Job drawing, mm, ordinate dimensions from the low corner. One solid piece. A direction names the side the tool comes from. Give positions to 0.01 mm unless a question says otherwise; leave off trailing zeros. Order: outer loops, then holes, each group sorted by start corner. A loop starts at its lowest first (then second) coordinate and runs counter-clockwise, first axis right, second up. Notation, with made-up numbers: M 13,-12 L 57,-12 A31 ccw 57,23 Z; hole C -30.5,-17.75 d2. An arc over 180 degrees is marked long. Put each result on its own line as item: value. Start each with the question number.
1) Drill centre lines: line 1 (Z direction, x = 32, y = 34); line 2 (Y direction, x = 9.5, z = 55.5); line 3 (Y direction, x = 50, z = 1.8). Where is each one in solid material? Low to high. Write a range as [from, to].
2) Tool access for the marked faces 1 and 2: list every direction of +Z, -Z, +X, -X, +Y, -Y with a clear straight run to the whole face (end or side of a thin tool).
3) Cut at B-B (y = 35.5). Write the cut outline in (x, z).
4) Pin check, flat tips, straight feed: pin 1 (12 mm diameter, centred on x = 75.5, z = 104.5, fed in from +Y); pin 2 (5.5 mm diameter, centred on y = 9, z = 115, fed in from -X); pin 3 (5.5 mm diameter, centred on y = 4.5, z = 114.5, fed in from +X). Stop position of each tip, or through.
5) Cut at D-D (y = 61). Write the cut outline in (x, z).
6) Cut at A-A (x = 75). Write the cut outline in (y, z).
7) Cut at C-C (z = 44.5). Write the cut outline in (x, y), and give its area (3 significant figures).
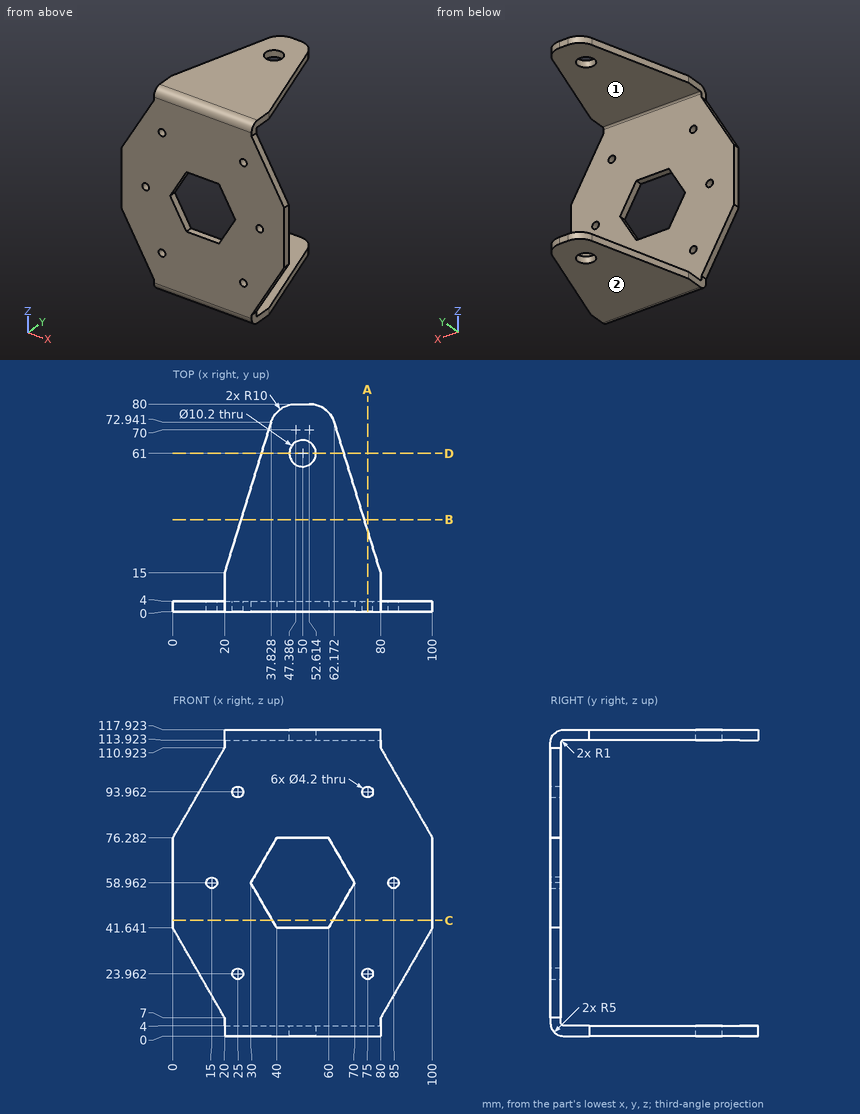
Solution:
1. line 1: [0, 4], [113.92, 117.92]
1. line 2: [0, 4]
1. line 3: [1.16, 55.9], [66.1, 80]
2. face 1: +X, -X, +Y
2. face 2: -Z, +X, -X, +Y, -Y
3. outline: M 26.31,0 L 73.69,0 L 73.69,4 L 26.31,4 Z; M 26.31,113.92 L 73.69,113.92 L 73.69,117.92 L 26.31,117.92 Z
4. pin 1: y = 4
4. pin 2: x = 20
4. pin 3: x = 80
5. outline: M 34.15,0 L 44.9,0 L 44.9,4 L 34.15,4 Z; M 34.15,113.92 L 44.9,113.92 L 44.9,117.92 L 34.15,117.92 Z; M 55.1,0 L 65.85,0 L 65.85,4 L 55.1,4 Z; M 55.1,113.92 L 65.85,113.92 L 65.85,117.92 L 55.1,117.92 Z
6. outline: M 0,5 A5 ccw 5,0 L 31.25,0 L 31.25,4 L 5,4 A1 cw 4,5 L 4,21.86 L 0,21.86 Z; M 0,26.06 L 4,26.06 L 4,91.86 L 0,91.86 Z; M 0,96.06 L 4,96.06 L 4,112.92 A1 cw 5,113.92 L 31.25,113.92 L 31.25,117.92 L 5,117.92 A5 ccw 0,112.92 Z
7. outline: M 0,0 L 38.35,0 L 38.35,4 L 0,4 Z; M 61.65,0 L 100,0 L 100,4 L 61.65,4 Z
7. area: 307 mm²
